Input: part model. Units: mm. Frame: model coordinates. Coordinates: 2 decimals unless noted, no trailing zeros. Loops run counter-clockwise (first coordinate to the right, second up) from the corner with the lowest first, then second, coordinate; pieces in that order, holes last. Notation, with made-up numbers: (2, 17) - (46, 17) arc R21 cw to (46, 35) - close; hole circle Ø7 at (64, 83.5). An arc over 180 degrees is marked (long way). Answer as CSV lines item,"result". Start each with the question number.
```python
from build123d import *

# Parameters (mm, degrees)
BOSS_EXTRUDE1_DEPTH = 2
SKETCH2_R           = 1
CUT_EXTRUDE1_DEPTH  = 132.191177295
CHAMFER1_SIZE       = 1.5
SKETCH3_W           = 16
SKETCH3_H           = 5
CUT_EXTRUDE2_DEPTH  = 132.191177295


with BuildPart() as part:
    # Sketch1 → Boss-Extrude1 (new body)
    with BuildSketch(Plane(origin=(0, 0, 0), x_dir=(1, 0, 0), z_dir=(0, 1, 0))):
        Polygon((-91.75, 91.75), (-91.75, -80.05), (-93.75, -80.05), (-93.75, -84.75), (-91.75, -84.75), (-91.75, -91.75), (-31.65, -91.75), (-31.65, -85.75), (21.65, -85.75), (21.65, -91.75), (91.75, -91.75), (91.75, -87.65), (86.75, -87.65), (86.75, -77.15), (91.75, -77.15), (91.75, 91.75), (18.65, 91.75), (18.65, 83.15), (-28.65, 83.15), (-28.65, 91.75), align=None)
    extrude(amount=BOSS_EXTRUDE1_DEPTH)

    # Sketch2 → Cut-Extrude1 (cut, through all)
    with BuildSketch(Plane.XZ):
        with Locations(Location((75, -75, 0), (0, 0, 270))):
            Circle(SKETCH2_R)
        with Locations(Location((-75, -75, 0), (0, 0, 270))):
            Circle(SKETCH2_R)
        with Locations(Location((-75, 75, 0), (0, 0, 270))):
            Circle(SKETCH2_R)
        with Locations(Location((75, 75, 0), (0, 0, 270))):
            Circle(SKETCH2_R)
        with Locations(Location((33.5, -38.5, 0), (0, 0, 270))):
            Circle(SKETCH2_R)
        with Locations(Location((33.5, 38.5, 0), (0, 0, 270))):
            Circle(SKETCH2_R)
        with Locations(Location((-43.5, -38.5, 0), (0, 0, 270))):
            Circle(SKETCH2_R)
        with Locations(Location((-43.5, 38.5, 0), (0, 0, 270))):
            Circle(SKETCH2_R)
    extrude(amount=-CUT_EXTRUDE1_DEPTH, mode=Mode.SUBTRACT)

    # Chamfer1
    chamfer1_edges = [part.edges().sort_by_distance(p)[0] for p in [
        (-75, 2, -74),
        (-75, 2, 76),
        (75, 2, 76),
        (33.5, 2, -37.5),
        (-43.5, 2, 39.5),
        (-43.5, 2, -37.5),
        (33.5, 2, 39.5),
        (75, 2, -74),
    ]]
    chamfer(chamfer1_edges, length=CHAMFER1_SIZE)

    # Sketch3 → Cut-Extrude2 (cut, through all)
    with BuildSketch(Plane.XZ):
        with Locations((-58.5, -87.5)):
            Rectangle(SKETCH3_W, SKETCH3_H)
    extrude(amount=-CUT_EXTRUDE2_DEPTH, mode=Mode.SUBTRACT)


solid = part.part
```
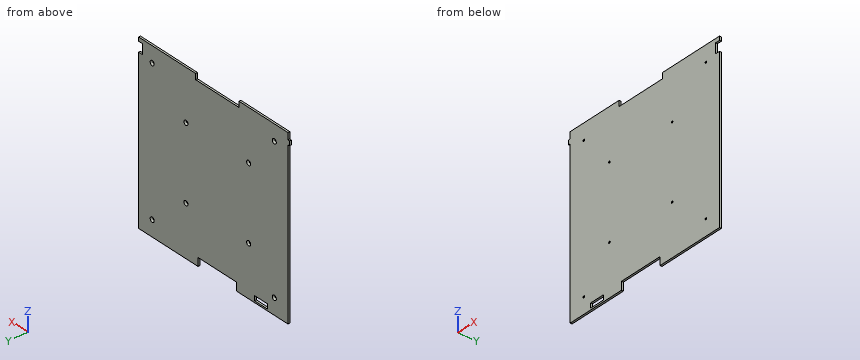
Item 1: Material intervals for probe 1 along X at (y, z) = (0.3, 38.5); probe 2 along X at (y, z) = (0.2, 75), sorted ascending.
Item 2: Section query A-A, the plane x = -58. Output: boundary loops of the cut face in (y, z).
Item 3: Section query C-C, the plane x = -6. Output: boundary loops of the cut face in (y, z).
Item 4: Contact query for flat-ended pins moving along their axis: P1, Ø0.6, axis at y = 0.5, z = 89, coming from the -X side; P2, Ø2.5, axis at x = -75, z = 75, coming from the +Y side; P3, Ø3, axis at x = 33.5, z = -38.5, coming from the +Y side. Output: stop coordinate, or through.
Item 5: Section query B-B, the plane y = 1.3. Give the number of separate pieces and of enclosed holes in the cut face, and give its area (3 significant figures).
Response values:
1,probe 1,"x = -91.75 to -44.5, -42.5 to 32.5, 34.5 to 91.75"
1,probe 2,"x = -91.75 to -76, -74 to 74, 76 to 91.75"
2,outline,"(0, -91.75) - (2, -91.75) - (2, -90) - (0, -90) - close; (0, -85) - (2, -85) - (2, 91.75) - (0, 91.75) - close"
3,outline,"(0, -83.15) - (2, -83.15) - (2, 85.75) - (0, 85.75) - close"
4,P1,"stops at x = -91.75"
4,P2,"stops at y = 0.75"
4,P3,"stops at y = 1"
5,separate pieces,"1"
5,enclosed holes,"9"
5,area,"32,700 mm²"
